Source: CAD feature listing. Evaluate the final solid. Frame: model axes, mm. Face numbers are marked on the shaded views. A direction names the side the tool comes from. Round coordinates to 2 decimals unless told otherwise and drop trailing zeros. Loops run counter-clockwise (first coordinate to the right, second up) from the corner with the lowest first, then second, coordinate; pieces in that order, holes last. Notation, with made-up numbers: M 14,21 L 73,21 A25 cw 73,48 Z; hole C -27.5,1 d1. An arc over 180 degrees is marked long. One line per item, written item: value.
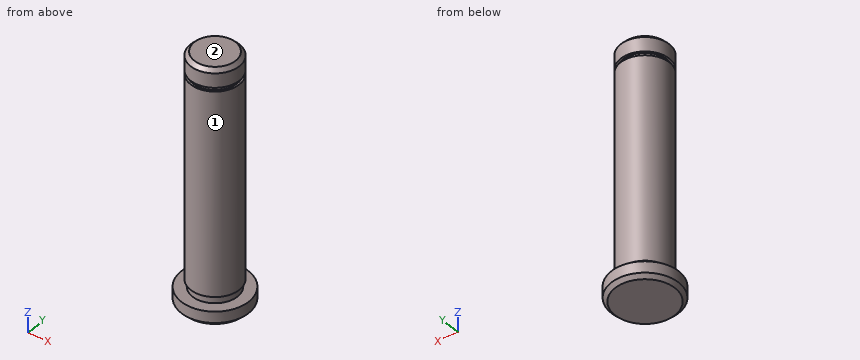
from build123d import *

# Parameters (mm, degrees)
SKETCH_1_R          = 9
EXTRUDE_1_DEPTH     = 4
SKETCH_2_R          = 6.5
EXTRUDE_2_DEPTH     = 62
SKETCH_4_OUTSIDE_W  = 34.148
SKETCH_4_OUTSIDE_H  = 34.148
SKETCH_4_OUTSIDE_R  = 6
CUT_EXTRUDE_1_DEPTH = 2
CUT_EXTRUDE_START   = -5.8
SKETCH_5_OUTSIDE_W  = 34.148
SKETCH_5_OUTSIDE_H  = 34.148
SKETCH_5_OUTSIDE_R  = 5.95
CUT_EXTRUDE_2_DEPTH = 1
CHAMFER_1_SIZE      = 1


with BuildPart() as part:
    # 草图1 → 凸台-拉伸1 (new body)
    with BuildSketch(Plane.XY):
        Circle(SKETCH_1_R)
    extrude(amount=EXTRUDE_1_DEPTH)

    # 草图2 → 凸台-拉伸2 (add)
    with BuildSketch(Plane.XY.offset(4)):
        Circle(SKETCH_2_R)
    extrude(amount=EXTRUDE_2_DEPTH)

    # 草图4 outside → 切除-拉伸1 (cut)
    with BuildSketch(Plane.XY.offset(4)):
        Rectangle(SKETCH_4_OUTSIDE_W, SKETCH_4_OUTSIDE_H)
        Circle(SKETCH_4_OUTSIDE_R, mode=Mode.SUBTRACT)
    extrude(amount=CUT_EXTRUDE_1_DEPTH, mode=Mode.SUBTRACT)

    # 草图5 outside → 切除-拉伸2 (cut)
    with BuildSketch(Plane.XY.offset(66).offset(CUT_EXTRUDE_START)):
        Rectangle(SKETCH_5_OUTSIDE_W, SKETCH_5_OUTSIDE_H)
        Circle(SKETCH_5_OUTSIDE_R, mode=Mode.SUBTRACT)
    extrude(amount=CUT_EXTRUDE_2_DEPTH, mode=Mode.SUBTRACT)

    # 倒角1
    chamfer_1_edges = [part.edges().sort_by_distance(p)[0] for p in [
        (-9, 0, 0),
        (-6.5, 0, 66),
    ]]
    chamfer(chamfer_1_edges, length=CHAMFER_1_SIZE)


solid = part.part
1. Ray query, line 1 (X direction, y = 0, z = 39.5); line 2 (Z direction, x = 1.5, y = 6.5); line 3 (Y direction, x = 2.5, z = 39.5). Return the intervals inside material, ascending. Write a range as [from, to].
Report:
line 1: x = [-6.5, 6.5]
line 2: z = [0, 4]
line 3: y = [-6, 6]
2. Section query C-C (z = 12.5). Return the cut outline in (x, y).
Report:
outline: C 0,0 d13
3. Section query A-A (x = 0). Return the cut outline in (y, z), and give its area (3 significant figures).
Report:
outline: M -9,1 L -8,0 L 8,0 L 9,1 L 9,4 L 6,4 L 6,6 L 6.5,6 L 6.5,60.2 L 5.95,60.2 L 5.95,61.2 L 6.5,61.2 L 6.5,65 L 5.5,66 L -5.5,66 L -6.5,65 L -6.5,61.2 L -5.95,61.2 L -5.95,60.2 L -6.5,60.2 L -6.5,6 L -6,6 L -6,4 L -9,4 Z
area: 873 mm2
4. Pin query (flat end, axial travel): pin 1 (3 mm diameter, centred on y = 6, z = 34.5, fed in from -X); pin 2 (2 mm diameter, centred on y = 2.5, z = 58.5, fed in from +X); pin 3 (1 mm diameter, centred on x = -0.5, y = 6.5, fed in from -Z); pin 4 (5 mm diameter, centred on x = 6, y = 5.5, fed in from +Z). Return the tip coordinate at first contact, or that it passes through.
Report:
pin 1: stops at x = -4.69
pin 2: stops at x = 6.32
pin 3: stops at z = 0
pin 4: stops at z = 65.86
5. Reachability of the marked faces 1 and 2 from +Z, -Z, +X, -X, +Y, -Y: full face, straight path, thin tool, end or side. Return the list, or none.
Report:
face 1: +Z
face 2: +Z, +X, -X, +Y, -Y
